Build history of the part. All positions in model axes, mm. A direction names the side the tool comes from. Round coordinates to 2 decimals unless told otherwise and drop trailing zeros. Order: outer loops, then holes, each group sorted by start corner. A loop starts at its lowest first (then second) coordinate and runs counter-clockwise, first axis right, second up. Notation, with made-up numbers: (41.25, 40) -> (100.25, 40) arc R12 cw to (100.25, 52) -> close; hole circle Ø6 at (-22, 53). An arc over 180 degrees is marked (long way). Answer as CSV lines item,"result". Start each with the question number.
```python
from build123d import *

# Parameters (mm, degrees)
BOSS_EXTRUDE1_DEPTH     = 65
CUT_EXTRUDE1_REACH      = 70.199
SKETCH2_R               = 1.374999977
SKETCH2_R_2             = 1.374999979
SKETCH2_R_3             = 1.374999935
SKETCH2_R_4             = 1.374999972
BOSS_EXTRUDE2_DEPTH     = 65
CUT_EXTRUDE3_REACH      = 70.199
CUT_EXTRUDE3_END_RADIUS = 9
SKETCH5_R               = 0.875
CUT_EXTRUDE4_REACH      = 76.384
CUT_EXTRUDE4_END_RADIUS = 15.5
SKETCH6_R               = 0.875
BOSS_EXTRUDE3_DEPTH     = 26
CUT_EXTRUDE7_DEPTH      = 69
SKETCH11_W              = 28.583211856
SKETCH11_H              = 6.5
CUT_EXTRUDE8_DEPTH      = 69


with BuildPart() as part:
    # Sketch1 → Boss-Extrude1 (new body)
    with BuildSketch(Plane.XY):
        with BuildLine():
            ThreePointArc((16.313540167, -7.607128711), (17.573328128, -3.895913051), (18, 0))
            Line((18, 0), (15.5, 0))
            ThreePointArc((15.5, 0), (15.13258811, -3.354814016), (14.047770699, -6.550583057))
            Line((14.047770699, -6.550583057), (16.313540167, -7.607128711))
        make_face()
        with BuildLine():
            Line((15.5, 0), (18, 0))
            ThreePointArc((18, 0), (17.9563329, 1.253039812), (17.82554347, 2.5))
            Line((17.82554347, 2.5), (15.297058541, 2.5))
            ThreePointArc((15.297058541, 2.5), (15.449181328, 1.254111761), (15.5, 0))
        make_face()
        with BuildLine():
            Line((-15.297058541, 2.5), (-17.82554347, 2.5))
            ThreePointArc((-17.82554347, 2.5), (-17.9563329, 1.253039812), (-18, 0))
            Line((-18, 0), (-15.5, 0))
            ThreePointArc((-15.5, 0), (-15.449181328, 1.254111761), (-15.297058541, 2.5))
        make_face()
        with BuildLine():
            Line((0, 0), (15.5, 0))
            ThreePointArc((15.5, 0), (15.449181328, 1.254111761), (15.297058541, 2.5))
            Line((15.297058541, 2.5), (-15.297058541, 2.5))
            ThreePointArc((-15.297058541, 2.5), (-15.449181328, 1.254111761), (-15.5, 0))
            Line((-15.5, 0), (0, 0))
        make_face()
        with BuildLine():
            ThreePointArc((-18, 0), (-17.573328128, -3.895913051), (-16.313540167, -7.607128711))
            Line((-16.313540167, -7.607128711), (-14.047770699, -6.550583057))
            ThreePointArc((-14.047770699, -6.550583057), (-15.13258811, -3.354814016), (-15.5, 0))
            Line((-15.5, 0), (-18, 0))
        make_face()
        with BuildLine():
            Line((15.5, 0), (18, 0))
            ThreePointArc((18, 0), (17.9563329, 1.253039812), (17.82554347, 2.5))
            Line((17.82554347, 2.5), (15.297058541, 2.5))
            ThreePointArc((15.297058541, 2.5), (15.449181328, 1.254111761), (15.5, 0))
        make_face()
        with BuildLine():
            Line((-15.297058541, 2.5), (-17.82554347, 2.5))
            ThreePointArc((-17.82554347, 2.5), (-17.9563329, 1.253039812), (-18, 0))
            Line((-18, 0), (-15.5, 0))
            ThreePointArc((-15.5, 0), (-15.449181328, 1.254111761), (-15.297058541, 2.5))
        make_face()
    extrude(amount=BOSS_EXTRUDE1_DEPTH)

    # Sketch2 → Cut-Extrude1 (cut, up to next)
    with BuildSketch(Plane(origin=(0, 2.5, 0), x_dir=(1, 0, 0), z_dir=(0, 1, 0)), mode=Mode.PRIVATE) as cut_extrude1_sk1:
        with Locations(Location((11.239474716, -3.394559676, 0), (0, 0, 270))):
            Circle(SKETCH2_R)
    cut_extrude1_tool1 = extrude(cut_extrude1_sk1.sketch, amount=-CUT_EXTRUDE1_REACH, mode=Mode.PRIVATE) & part.part
    # Sketch2 → Cut-Extrude1 (cut, up to next)
    with BuildSketch(Plane(origin=(0, 2.5, 0), x_dir=(1, 0, 0), z_dir=(0, 1, 0)), mode=Mode.PRIVATE) as cut_extrude1_sk2:
        with Locations(Location((-11.760472903, -3.443135131, 0), (0, 0, 270))):
            Circle(SKETCH2_R_2)
    cut_extrude1_tool2 = extrude(cut_extrude1_sk2.sketch, amount=-CUT_EXTRUDE1_REACH, mode=Mode.PRIVATE) & part.part
    # Sketch2 → Cut-Extrude1 (cut, up to next)
    with BuildSketch(Plane(origin=(0, 2.5, 0), x_dir=(1, 0, 0), z_dir=(0, 1, 0)), mode=Mode.PRIVATE) as cut_extrude1_sk3:
        with Locations(Location((11.361823253, -61.347443071, 0), (0, 0, 270))):
            Circle(SKETCH2_R_3)
    cut_extrude1_tool3 = extrude(cut_extrude1_sk3.sketch, amount=-CUT_EXTRUDE1_REACH, mode=Mode.PRIVATE) & part.part
    # Sketch2 → Cut-Extrude1 (cut, up to next)
    with BuildSketch(Plane(origin=(0, 2.5, 0), x_dir=(1, 0, 0), z_dir=(0, 1, 0)), mode=Mode.PRIVATE) as cut_extrude1_sk4:
        with Locations(Location((-11.637978285, -61.443005778, 0), (0, 0, 270))):
            Circle(SKETCH2_R_4)
    cut_extrude1_tool4 = extrude(cut_extrude1_sk4.sketch, amount=-CUT_EXTRUDE1_REACH, mode=Mode.PRIVATE) & part.part
    add(cut_extrude1_tool1.solids().sort_by_distance((11.239475, 2.5, 3.39456))[0], mode=Mode.SUBTRACT)
    add(cut_extrude1_tool2.solids().sort_by_distance((-11.760473, 2.5, 3.443135))[0], mode=Mode.SUBTRACT)
    add(cut_extrude1_tool3.solids().sort_by_distance((11.361823, 2.5, 61.347443))[0], mode=Mode.SUBTRACT)
    add(cut_extrude1_tool4.solids().sort_by_distance((-11.637978, 2.5, 61.443006))[0], mode=Mode.SUBTRACT)

    # Sketch3 → Boss-Extrude2 (add)
    with BuildSketch(Plane.XY.offset(65)):
        with BuildLine():
            Line((-9, 0), (-9, -6))
            Line((-9, -6), (-8.485281374, -6))
            ThreePointArc((-8.485281374, -6), (-5.196152423, -1.651530772), (0, 0))
            Line((0, 0), (-9, 0))
        make_face()
        with BuildLine():
            ThreePointArc((0, 0), (5.196152423, -1.651530772), (8.485281374, -6))
            Line((8.485281374, -6), (9, -6))
            Line((9, -6), (9, 0))
            Line((9, 0), (0, 0))
        make_face()
    extrude(amount=-BOSS_EXTRUDE2_DEPTH)

    # Cut-Extrude3: up to this cylinder (the profile starts outside it)
    cut_extrude3_end = Plane(origin=(0, -9, 2), z_dir=(0, 0, 1)) * Cylinder(CUT_EXTRUDE3_END_RADIUS, 159.398, mode=Mode.PRIVATE)
    # Sketch5 → Cut-Extrude3 (cut, up to the surface)
    with BuildSketch(Plane(origin=(0, 2.5, 0), x_dir=(1, 0, 0), z_dir=(0, 1, 0)), mode=Mode.PRIVATE) as cut_extrude3_sk1:
        with Locations(Location((-5.7, -2, 0), (0, 0, 270))):
            Circle(SKETCH5_R)
    cut_extrude3_tool1 = extrude(cut_extrude3_sk1.sketch, amount=-CUT_EXTRUDE3_REACH, mode=Mode.PRIVATE) - cut_extrude3_end
    add(cut_extrude3_tool1.solids().sort_by_distance((-5.7, 2.5, 2))[0], mode=Mode.SUBTRACT)
    # Sketch5 → Cut-Extrude3 (cut, up to the surface)
    with BuildSketch(Plane(origin=(0, 2.5, 0), x_dir=(1, 0, 0), z_dir=(0, 1, 0)), mode=Mode.PRIVATE) as cut_extrude3_sk2:
        with Locations(Location((5.7, -2, 0), (0, 0, 270))):
            Circle(SKETCH5_R)
    cut_extrude3_tool2 = extrude(cut_extrude3_sk2.sketch, amount=-CUT_EXTRUDE3_REACH, mode=Mode.PRIVATE) - cut_extrude3_end
    add(cut_extrude3_tool2.solids().sort_by_distance((5.7, 2.5, 2))[0], mode=Mode.SUBTRACT)

    # Cut-Extrude4: up to this cylinder (the profile starts outside it)
    cut_extrude4_end = Plane(origin=(0, 0, 32.5), z_dir=(0, 0, -1)) * Cylinder(CUT_EXTRUDE4_END_RADIUS, 229.768, mode=Mode.PRIVATE)
    # Sketch6 → Cut-Extrude4 (cut, up to the surface)
    with BuildSketch(Plane(origin=(-17.726539554, -3.125667198, 0), x_dir=(0, 0, -1), z_dir=(-0.984807753012208, -0.17364817766693072, 0)), mode=Mode.PRIVATE) as cut_extrude4_sk1:
        with Locations(Location((-55, -1.057392522, 0), (0, 0, 90))):
            Circle(SKETCH6_R)
    cut_extrude4_tool1 = extrude(cut_extrude4_sk1.sketch, amount=-CUT_EXTRUDE4_REACH, mode=Mode.PRIVATE) - cut_extrude4_end
    # Sketch6 → Cut-Extrude4 (cut, up to the surface)
    with BuildSketch(Plane(origin=(-17.726539554, -3.125667198, 0), x_dir=(0, 0, -1), z_dir=(-0.984807753012208, -0.17364817766693072, 0)), mode=Mode.PRIVATE) as cut_extrude4_sk2:
        with Locations(Location((-10, -1.057392522, 0), (0, 0, 90))):
            Circle(SKETCH6_R)
    cut_extrude4_tool2 = extrude(cut_extrude4_sk2.sketch, amount=-CUT_EXTRUDE4_REACH, mode=Mode.PRIVATE) - cut_extrude4_end
    cut_extrude4 = cut_extrude4_tool1.solids().sort_by_distance((-17.910154, -2.084339, 55))[0] + cut_extrude4_tool2.solids().sort_by_distance((-17.910154, -2.084339, 10))[0]
    add(cut_extrude4, mode=Mode.SUBTRACT)

    # Mirror1: Cut-Extrude4 across plane
    add(cut_extrude4.mirror(Plane(origin=(0, 0, 0), x_dir=(0, 0, 1), z_dir=(1, 0, 0))), mode=Mode.SUBTRACT)

    # Sketch8 → Boss-Extrude3 (add, symmetric)
    with BuildSketch(Plane.XY.offset(32.5)):
        with BuildLine():
            Line((-14.291605928, -6), (-9, -6))
            Line((-9, -6), (-9, 0))
            Line((-9, 0), (-15.5, 0))
            ThreePointArc((-15.5, 0), (-15.194898682, -3.060237582), (-14.291605928, -6))
        make_face()
        with BuildLine():
            Line((9, 0), (9, -6))
            Line((9, -6), (14.291605928, -6))
            ThreePointArc((14.291605928, -6), (15.194898682, -3.060237582), (15.5, 0))
            Line((15.5, 0), (9, 0))
        make_face()
    extrude(amount=BOSS_EXTRUDE3_DEPTH, both=True)

    # Sketch9 → Cut-Extrude7 (cut)
    with BuildSketch(Plane.XY.offset(65)):
        with BuildLine():
            ThreePointArc((-14.047770699, -6.550583057), (-14.172362271, -6.276475737), (-14.291605928, -6))
            Line((-14.291605928, -6), (-16.970562748, -6))
            ThreePointArc((-16.970562748, -6), (-16.661440286, -6.811490851), (-16.313540167, -7.607128711))
            Line((-16.313540167, -7.607128711), (-14.047770699, -6.550583057))
        make_face()
        with BuildLine():
            Line((16.970562748, -6), (14.291605928, -6))
            ThreePointArc((14.291605928, -6), (14.172362271, -6.276475737), (14.047770699, -6.550583057))
            Line((14.047770699, -6.550583057), (16.313540167, -7.607128711))
            ThreePointArc((16.313540167, -7.607128711), (16.661440286, -6.811490851), (16.970562748, -6))
        make_face()
    extrude(amount=-CUT_EXTRUDE7_DEPTH, mode=Mode.SUBTRACT)

    # Sketch11 → Cut-Extrude8 (cut)
    with BuildSketch(Plane(origin=(0, 0, 0), x_dir=(-1, 0, 0), z_dir=(0, -1, 0))):
        with Locations((0, -61.75)):
            Rectangle(SKETCH11_W, SKETCH11_H)
        with Locations((0, -3.25)):
            Rectangle(SKETCH11_W, SKETCH11_H)
    extrude(amount=CUT_EXTRUDE8_DEPTH, mode=Mode.SUBTRACT)


solid = part.part
```
Q1. Slice it at D-D, the plane x = 5.7. Write the cut outline in (y, z) (3 decimals).
Q2. Which spindle directions (+Z, -Z, +X, -X, +Y, -Y) get a long thin tool onto all of the face, cutting with end or side? Do faces 3 (the face through (15.41, -1.65, 55.01)), 4 (the face through (-10, -2, 6.5)), 5 (the face through (-11, -2, 58.5)). Say none if no direction does.
Q3. Probe L1, parallel to Z at x = -12.5, y = 1.25; L2, parallel to Y at x = 0.5, z = 40.5; L3, parallel to X at y = 0.5, z = 21. List the from-to ranges inside material, lowest first.
Q4. Slice it at B-B, the plane x = 13.5. Write the cut outline in (y, z).
Q5. Slice it at C-C, the plane z = 25. Write the cut outline in (x, y), plus the area to 3 significant figures.
Q6. Slice it at A-A, the plane y = -4.75. Write the cut outline in (x, z), plus the area to 3 significant figures.
Q7. Two-plate mould, pull along X, no slides. Class faces 1 (the face through (13, -6, 33)), 2 (the face through (16.657, -1.748, 55.868)): +X half, -X half, draft (parallel to the pull), parting line (faces both ways), or undercut.
Q8. Flat gauge pins, fed straight in: pin 1 Ø1 at (x, y) = (10, -5) entering from -Z; pin 2 Ø4.5 at (x, z) = (11.36, 61.35) entering from -Y; pin 3 Ø4 at (y, z) = (-4.5, 51) entering from -X; pin 4 Ø3.5 at (x, z) = (-11.76, 3.44) entering from +Y. Where does each tip first touch, or does it go through?
Solutions:
1,outline,"(-2.035, 6.5) -> (0, 6.5) -> (0, 2.875) -> (2.5, 2.875) -> (2.5, 65) -> (0, 65) -> (0, 58.5) -> (-2.035, 58.5) -> close; (0, 0) -> (2.5, 0) -> (2.5, 1.125) -> (0, 1.125) -> close"
2,face 3,"none"
2,face 4,"-Z"
2,face 5,"+Z"
3,L1,"z = 0 to 2.28, 4.6 to 60.37, 62.51 to 65"
3,L2,"y = -0.01 to 2.5"
3,L3,"x = -17.99 to 17.99"
4,outline,"(-6, 6.5) -> (0, 6.5) -> (0, 0) -> (2.5, 0) -> (2.5, 65) -> (0, 65) -> (0, 58.5) -> (-6, 58.5) -> close"
5,outline,"(-17.83, 2.5) arc R18 ccw to (-16.97, -6) -> (-8.49, -6) arc R9 cw to (8.49, -6) -> (16.97, -6) arc R18 ccw to (17.83, 2.5) -> close"
5,area,"227 mm2"
6,outline,"(-17.36, 0) -> (-14.75, 0) -> (-14.75, 6.5) -> (-7.93, 6.5) -> (-7.93, 58.5) -> (-14.75, 58.5) -> (-14.75, 65) -> (-17.36, 65) -> close; (7.93, 6.5) -> (14.75, 6.5) -> (14.75, 0) -> (17.36, 0) -> (17.36, 65) -> (14.75, 65) -> (14.75, 58.5) -> (7.93, 58.5) -> close"
6,area,"1,050 mm2"
7,face 1,"draft"
7,face 2,"undercut"
8,pin 1,"stops at z = 6.5"
8,pin 2,"stops at y = 0"
8,pin 3,"stops at x = -17.83"
8,pin 4,"stops at y = 2.5"
